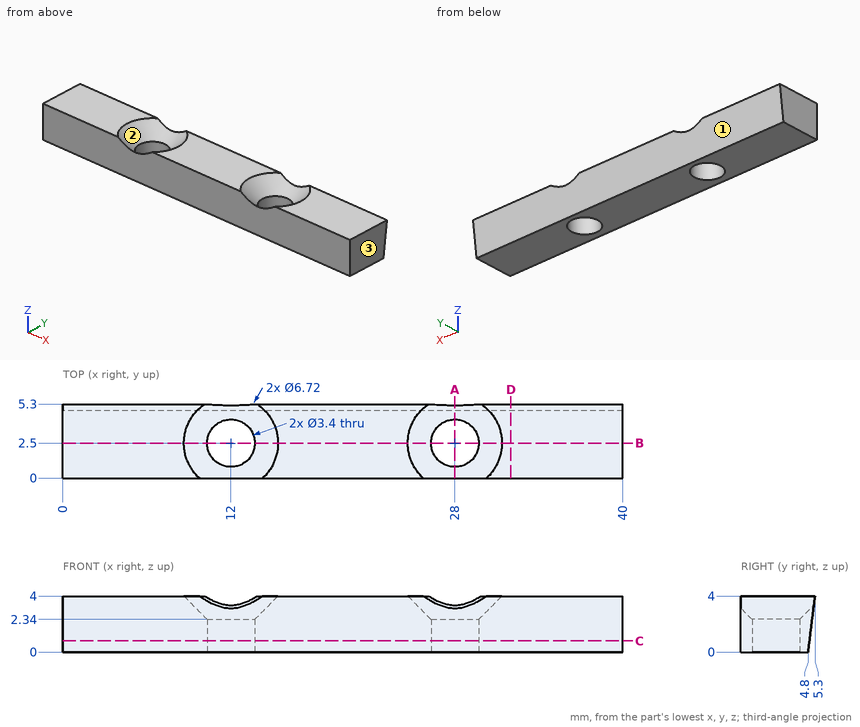
For this review, use the dimensioned drawing (mm, ordinates from the lowest corner) and the shaded views. Coordinates: 2 decimals unless noted, no trailing zeros. Loops run counter-clockwise (first coordinate to the right, second up) from the corner with the lowest first, then second, coordinate; pieces in that order, holes last. Notation, with made-up numbers: (-15, 21.25) -> (26, 21.25) arc R22 ccw to (26, 34.25) -> close; hole circle Ø1 at (34, 70). An arc over 180 degrees is marked (long way). Return JSON: item names as keys, results as strings. Group by question number.
(1) To check wall thickness, follow L1, parallel to X at y = 2.5, z = 1; L2, parallel to X at y = 1.4, z = 1.4; L3, parallel to Y at x = 12, z = 1.8 (3 decimals). State the ranges of each line that lie inside material, in increasing order.
(2) Consider section C-C, the plane z = 0.8. Give the boundary of the cut face in (x, y).
(3) Consider section B-B, the plane y = 2.5. Give the boundary of the cut face in (x, z), plus the area to 3 significant figures.
(4) Mouldability with a two-part tool opening along X and no side actions: class the marked faces 1, 2 and 3 as pulls with the +X half, pulls with the -X half, needs draft (parallel to the pull), parting line crosses it, or undercut.
(5) Consider section A-A, the plane x = 28. Give the boundary of the cut face in (y, z), plus the area to 3 significant figures.
(6) For pin 1 Ø3 at (x, y) = (28, 2.5) entering from -Z, flat-tipped, find the tip position at first contact; note if it passes through.
(7) Consider section D-D, the plane x = 32. Give the boundary of the cut face in (y, z).
Results below:
{
 "1": {"L1": "x = 0 to 10.3, 13.7 to 26.3, 29.7 to 40", "L2": "x = 0 to 10.7, 13.3 to 26.7, 29.3 to 40", "L3": "y = 0 to 0.8, 4.2 to 5.025"},
 "2": {"outline": "(0, 0) -> (40, 0) -> (40, 4.9) -> (0, 4.9) -> close; hole circle Ø3.4 at (12, 2.5); hole circle Ø3.4 at (28, 2.5)"},
 "3": {"outline": "(0, 0) -> (10.3, 0) -> (10.3, 2.34) -> (8.64, 4) -> (0, 4) -> close; (13.7, 0) -> (26.3, 0) -> (26.3, 2.34) -> (24.64, 4) -> (15.36, 4) -> (13.7, 2.34) -> close; (29.7, 0) -> (40, 0) -> (40, 4) -> (31.36, 4) -> (29.7, 2.34) -> close", "area": "127 mm2"},
 "4": {"face 1": "needs draft", "face 2": "undercut", "face 3": "pulls with the +X half"},
 "5": {"outline": "(0, 0) -> (0.8, 0) -> (0.8, 2.34) -> (0, 3.14) -> close; (4.2, 0) -> (4.8, 0) -> (5.22, 3.36) -> (4.2, 2.34) -> close", "area": "4.39 mm2"},
 "6": {"pin 1": "passes through"},
 "7": {"outline": "(0, 0) -> (4.8, 0) -> (5.3, 4) -> (0, 4) -> close"}
}
